Can you work these out from the model? Positions are in its coordinate system, mm. Face numbers are marked on the shaded views. Coordinates: 2 decimals unless noted, no trailing zeros. Loops run counter-clockwise (first coordinate to the right, second up) from the corner with the lowest first, then second, coordinate; pieces in that order, holes last. Notation, with made-up numbers: (-10.5, 36) -> (32.5, 36) arc R17 ccw to (32.5, 66) -> close; hole circle Ø4 at (-10, 80.5). An arc over 180 degrees is marked (long way). Use one line per item in the form item = value. Start each with the question number.
(1) Imagine slicing it at A-A (y = 5). List the corners of the cut face in (x, z) for me, plus the area to 3 significant figures.
(2) I need wall thicknesses on line 1 (X direction, y = -8.5, z = 10.25); line 2 (Y direction, x = -23, z = 8.5); line 3 (Z direction, x = 37.5, y = -4). Which ranges of each line are inside material? Lowest first, please. Write a range as [from, to].
(3) Imagine slicing it at D-D (y = -9). List the corners of the cut face in (x, z) for me, plus the area to 3 significant figures.
(4) Imagine slicing it at B-B (z = 8). List the corners of the cut face in (x, y) for me, plus the area to 3 significant figures.
(5) I'm going to push flat-ended pins straight in: pin 1 (6 mm diameter, centred on y = -16, z = 14.5, fed in from +X); pin 2 (8 mm diameter, centred on y = 13, z = 14.5, fed in from +X); pin 3 (1.5 mm diameter, centred on x = -15.5, y = 29.5, fed in from +Z); pin 4 (2.5 mm diameter, centred on x = 43.5, z = 14, fed in from +Y). Where does each tip first touch, or does it pass through?
(6) Imagine slicing it at C-C (x = 36). List the corners of the cut face in (y, z) for me, plus the area to 3 significant figures.
(7) Thinking about a two-plate mould opening in X: for the marked faces 1, 2 and 3, which applies, released by +X, released by -X, zero draft, split by the parting line, or undercut?
```python
from build123d import *

# Parameters (mm, degrees)
SKETCH1_W           = 91
SKETCH1_H           = 62
BOSS_EXTRUDE1_DEPTH = 3
SKETCH2_W           = 91
SKETCH2_H           = 62
SKETCH2_W_2         = 85
SKETCH2_H_2         = 56
BOSS_EXTRUDE2_DEPTH = 15.5
FILLET1_R           = 5
SKETCH3_W           = 3
SKETCH3_H           = 15.9
SKETCH3_H_2         = 13.8
CUT_EXTRUDE2_DEPTH  = 15.5
SKETCH4_W           = 8.94
SKETCH4_H           = 3
SKETCH4_W_2         = 6.5
CUT_EXTRUDE3_DEPTH  = 3.5
SKETCH5_W           = 14.75
SKETCH5_H           = 3
CUT_EXTRUDE4_DEPTH  = 5.65
SKETCH6_W           = 0.75
SKETCH6_H           = 15
CUT_EXTRUDE5_DEPTH  = 3


with BuildPart() as part:
    # Sketch1 → Boss-Extrude1 (new body)
    with BuildSketch(Plane.XY):
        Rectangle(SKETCH1_W, SKETCH1_H)
    extrude(amount=BOSS_EXTRUDE1_DEPTH)

    # Sketch2 → Boss-Extrude2 (add)
    with BuildSketch(Plane.XY.offset(3)):
        Rectangle(SKETCH2_W, SKETCH2_H)
        Rectangle(SKETCH2_W_2, SKETCH2_H_2, mode=Mode.SUBTRACT)
    extrude(amount=BOSS_EXTRUDE2_DEPTH)

    # Fillet1
    fillet1_edges = [part.edges().sort_by_distance(p)[0] for p in [
        (45.5, -31, 9.25),
        (-45.5, -31, 9.25),
        (-45.5, 31, 9.25),
        (45.5, 31, 9.25),
    ]]
    fillet(fillet1_edges, radius=FILLET1_R)

    # Sketch3 → Cut-Extrude2 (cut)
    with BuildSketch(Plane.XY.offset(18.5)):
        with Locations((44, -18)):
            Rectangle(SKETCH3_W, SKETCH3_H)
        with Locations((44, 0.75)):
            Rectangle(SKETCH3_W, SKETCH3_H_2)
        with Locations((44, 18.75)):
            Rectangle(SKETCH3_W, SKETCH3_H_2)
    extrude(amount=-CUT_EXTRUDE2_DEPTH, mode=Mode.SUBTRACT)

    # Sketch4 → Cut-Extrude3 (cut)
    with BuildSketch(Plane.XY.offset(18.5)):
        with Locations((-31.3, 29.5)):
            Rectangle(SKETCH4_W, SKETCH4_H)
        with Locations((-16.5, 29.5)):
            Rectangle(SKETCH4_W_2, SKETCH4_H)
        with Locations((-3, 29.5)):
            Rectangle(SKETCH4_W_2, SKETCH4_H)
    extrude(amount=-CUT_EXTRUDE3_DEPTH, mode=Mode.SUBTRACT)

    # Sketch5 → Cut-Extrude4 (cut)
    with BuildSketch(Plane.XY.offset(18.5)):
        with Locations((1.125, 29.5)):
            Rectangle(SKETCH5_W, SKETCH5_H)
    extrude(amount=-CUT_EXTRUDE4_DEPTH, mode=Mode.SUBTRACT)

    # Sketch6 → Cut-Extrude5 (cut)
    with BuildSketch(Plane(origin=(0, 0, 0), x_dir=(-1, 0, 0), z_dir=(0, 0, -1))):
        with Locations((10.125, 0)):
            Rectangle(SKETCH6_W, SKETCH6_H)
    extrude(amount=-CUT_EXTRUDE5_DEPTH, mode=Mode.SUBTRACT)


solid = part.part
```
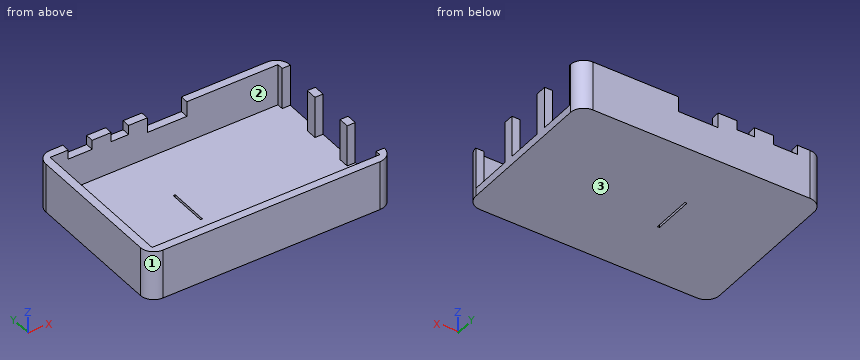
Worked out:
q1.outline = (-45.5, 0) -> (-10.5, 0) -> (-10.5, 3) -> (-42.5, 3) -> (-42.5, 18.5) -> (-45.5, 18.5) -> close; (-9.75, 0) -> (45.5, 0) -> (45.5, 3) -> (-9.75, 3) -> close
q1.area = 317 mm2
q2.line_1 = [-45.5, -42.5], [42.5, 45.5]
q2.line_2 = [-31, -28], [28, 31]
q2.line_3 = [0, 3]
q3.outline = (-45.5, 0) -> (45.5, 0) -> (45.5, 18.5) -> (42.5, 18.5) -> (42.5, 3) -> (-42.5, 3) -> (-42.5, 18.5) -> (-45.5, 18.5) -> close
q3.area = 366 mm2
q4.outline = (-45.5, -26) arc R5 ccw to (-40.5, -31) -> (40.5, -31) arc R5 ccw to (45.5, -26) -> (45.5, -25.95) -> (42.5, -25.95) -> (42.5, -28) -> (-42.5, -28) -> (-42.5, 28) -> (42.5, 28) -> (42.5, 25.65) -> (45.5, 25.65) -> (45.5, 26) arc R5 ccw to (40.5, 31) -> (-40.5, 31) arc R5 ccw to (-45.5, 26) -> close; (42.5, -10.05) -> (45.5, -10.05) -> (45.5, -6.15) -> (42.5, -6.15) -> close; (42.5, 7.65) -> (45.5, 7.65) -> (45.5, 11.85) -> (42.5, 11.85) -> close
q4.area = 730 mm2
q5.pin_1 = -42.5
q5.pin_2 = 45.5
q5.pin_3 = 15
q5.pin_4 = 30.68
q6.outline = (-31, 0) -> (31, 0) -> (31, 18.5) -> (28, 18.5) -> (28, 3) -> (-28, 3) -> (-28, 18.5) -> (-31, 18.5) -> close
q6.area = 279 mm2
q7.face_1 = released by -X
q7.face_2 = undercut
q7.face_3 = zero draft
